from build123d import *

# Parameters (mm, degrees)
F1_W     = 56
F1_H     = 69
F4_DEPTH = 5
F2_W     = 8
F2_H     = 20
F5_DEPTH = 4
F3_R     = 0.889
F3_R_2   = 1.143
F3_R_3   = 2.9
F6_DEPTH = 5.001


with BuildPart() as f4:
    # F1 (on Front) → F4 (new body)
    with BuildSketch(Plane.XZ):
        with Locations((-0.375, 2)):
            Rectangle(F1_W, F1_H)
    extrude(amount=F4_DEPTH)

    # F2 (on Front) → F5 (cut)
    with BuildSketch(Plane.XZ):
        Polygon((-20.875, 12.5), (-20.875, 2.5), (-12.875, 2.5), (-12.875, 22.5), (-20.875, 22.5), align=None)
        with Locations((-16.875, -18.5)):
            Rectangle(F2_W, F2_H)
        Polygon((20.125, 12.5), (20.125, 22.5), (12.125, 22.5), (12.125, 2.5), (20.125, 2.5), align=None)
        with Locations((16.125, -18.5)):
            Rectangle(F2_W, F2_H)
    extrude(amount=F5_DEPTH, mode=Mode.SUBTRACT)

    # F3 (on Front) → F6 (cut, through all)
    with BuildSketch(Plane.XZ):
        with Locations((-25.875, 18.5)):
            Circle(F3_R)
        with Locations((-25.875, 6.5)):
            Circle(F3_R)
        with Locations((-8.875, 18.5)):
            Circle(F3_R)
        with Locations((-8.875, 6.5)):
            Circle(F3_R)
        with Locations((-8.875, -12.5)):
            Circle(F3_R)
        with Locations((-25.875, -12.5)):
            Circle(F3_R)
        with Locations((-25.875, -24.5)):
            Circle(F3_R)
        with Locations((-8.875, -24.5)):
            Circle(F3_R)
        with Locations((-0.375, -30)):
            Circle(F3_R_2)
        with Locations((-25.375, -29.5)):
            Circle(F3_R_2)
        with Locations((-0.375, -3)):
            Circle(F3_R_3)
        with Locations((-25.375, 33.5)):
            Circle(F3_R_2)
        with Locations((8.125, 18.5)):
            Circle(F3_R)
        with Locations((8.125, 6.5)):
            Circle(F3_R)
        with Locations((25.125, 18.5)):
            Circle(F3_R)
        with Locations((24.625, 33.5)):
            Circle(F3_R_2)
        with Locations((8.125, -12.5)):
            Circle(F3_R)
        with Locations((8.125, -24.5)):
            Circle(F3_R)
        with Locations((25.125, -12.5)):
            Circle(F3_R)
        with Locations((25.125, -24.5)):
            Circle(F3_R)
        with Locations((24.625, -29.5)):
            Circle(F3_R_2)
        with Locations((25.125, 6.5)):
            Circle(F3_R)
        with Locations((-20.375, 33.5)):
            Circle(F3_R_2)
        with Locations((19.625, 33.5)):
            Circle(F3_R_2)
    extrude(amount=F6_DEPTH, mode=Mode.SUBTRACT)


solid = f4.part
Geometry check sheet. Reference: the model listing, model coordinates, mm. A direction names the side the tool comes from. Give positions to 0.01 mm unless a question says otherwise; leave off trailing zeros. Write each loop counter-clockwise with the first axis right and the second up, starting at its lowest first coordinate (ties: lowest second). Pieces come first, ordered by that corner, then holes.
1) Cross-section at B-B (z = 8.5). Record the boundary of the cut face in (x, y) (3 decimals).
Values follow:
outline: (-28.375, -5) - (27.625, -5) - (27.625, 0) - (20.125, 0) - (20.125, -4) - (12.125, -4) - (12.125, 0) - (-12.875, 0) - (-12.875, -4) - (-20.875, -4) - (-20.875, 0) - (-28.375, 0) - close
2) Cross-section at A-A (z = 33.5). Record the boundary of the cut face in (x, y) (3 decimals), plus the area to 3 significant figures.
Values follow:
outline: (-28.375, -5) - (-26.518, -5) - (-26.518, 0) - (-28.375, 0) - close; (-24.232, -5) - (-21.518, -5) - (-21.518, 0) - (-24.232, 0) - close; (-19.232, -5) - (18.482, -5) - (18.482, 0) - (-19.232, 0) - close; (20.768, -5) - (23.482, -5) - (23.482, 0) - (20.768, 0) - close; (25.768, -5) - (27.625, -5) - (27.625, 0) - (25.768, 0) - close
area: 234 mm2
3) Go/stop test with a flat-tipped pin: pin 1 Ø1.4 at (x, z) = (-25.375, 33.5) entering from -Y. Record where the tip stops, or that it passes through.
Values follow:
pin 1: passes through
4) Cross-section at D-D (z = -2). Record the boundary of the cut face in (x, y) (3 decimals), plus the area to 3 significant figures.
Values follow:
outline: (-28.375, -5) - (-3.097, -5) - (-3.097, 0) - (-28.375, 0) - close; (2.347, -5) - (27.625, -5) - (27.625, 0) - (2.347, 0) - close
area: 253 mm2
5) Set-up check for faces 1 (the face through (-17, -4, -18)), 2 (the face through (-25.4, -2.46, -23.75)): record each of +Z, -Z, +X, -X, +Y, -Y from which the full face is reachable in a straight line by a thin tool's end or side.
Values follow:
face 1: +Y
face 2: +Y, -Y
6) Thickness scan on line 1 (X direction, y = -2.3, z = 14) (3 decimals); line 2 (X direction, y = -1.1, z = 33.5) (3 decimals); line 3 (Z direction, x = -13.5, y = -0.9). Record the ranges inside material, lowest first.
Values follow:
line 1: x = -28.375 to -20.875, -12.875 to 12.125, 20.125 to 27.625
line 2: x = -28.375 to -26.518, -24.232 to -21.518, -19.232 to 18.482, 20.768 to 23.482, 25.768 to 27.625
line 3: z = -32.5 to -28.5, -8.5 to 2.5, 22.5 to 36.5
7) Release check for a two-part mould opening along X. For faces 3 (the face through (-1, 0, 2)), 4 (the face through (-25.054, -2.465, 6.16)), 5 (the face through (-28.375, -2, 2)) record: released by +X, released by -X, zero draft, split by the parting line, or undercut.
Values follow:
face 3: zero draft
face 4: undercut
face 5: released by -X
8) Cross-section at C-C (x = -20). Record the boundary of the cut face in (y, z), plus the area to 3 significant figures.
Values follow:
outline: (-5, -32.5) - (0, -32.5) - (0, -28.5) - (-4, -28.5) - (-4, -8.5) - (0, -8.5) - (0, 2.5) - (-4, 2.5) - (-4, 22.5) - (0, 22.5) - (0, 32.42) - (-5, 32.42) - close; (-5, 34.58) - (0, 34.58) - (0, 36.5) - (-5, 36.5) - close
area: 174 mm2
